Verification items for the finished model (mm, model axes). Face numbers are marked on the shaded views. Give positions to 0.01 mm unless a question says otherwise; leave off trailing zeros. Write each loop counter-clockwise with the first axis right and the second up, starting at its lowest first coordinate (ties: lowest second). Pieces come first, ordered by that corner, then holes.
from build123d import *

# Parameters (mm, degrees)
SKETCH_1_W      = 11
SKETCH_1_H      = 6
SKETCH_1_R      = 1.5
EXTRUDE_1_DEPTH = 2
CHAMFER_1_SIZE  = 1


with BuildPart() as part:
    # Эскиз1 → Бобышка-Вытянуть1 (new body)
    with BuildSketch(Plane(origin=(0, 0, 0), x_dir=(0, 0, -1), z_dir=(1, 0, 0))):
        with Locations((-5.5, 3)):
            Rectangle(SKETCH_1_W, SKETCH_1_H)
        with Locations((-2.5, 3)):
            Circle(SKETCH_1_R, mode=Mode.SUBTRACT)
    extrude(amount=EXTRUDE_1_DEPTH)

    # Фаска1
    chamfer_1_edges = [part.edges().sort_by_distance(p)[0] for p in [
        (0, 3, 4),
    ]]
    chamfer(chamfer_1_edges, length=CHAMFER_1_SIZE - 0.0001)  # a hair under: the kernel refuses the full size


solid = part.part
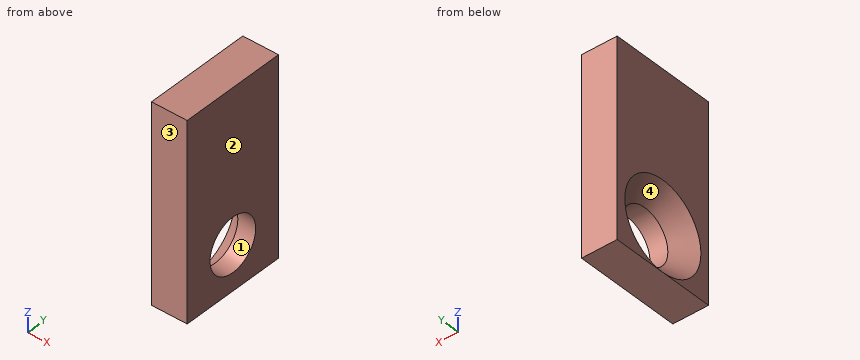
Item 1: Depth check by flat-ended pin: pin 1 (1.8 mm diameter, centred on y = 3, z = 2.5, fed in from +X). Enter the tip coordinate at first touch or a pass-through.
Answer key:
pin 1: passes through
Item 2: Sectioned sample at B-B on z = 2.5. Record the cut outline in (x, y), then the cut area to 3 significant figures.
Answer key:
outline: (0, 0) - (2, 0) - (2, 1.5) - (1, 1.5) - (0, 0.5) - close; (0, 5.5) - (1, 4.5) - (2, 4.5) - (2, 6) - (0, 6) - close
area: 5.00 mm2
Item 3: Sectioned sample at C-C on x = 1.15. Record the cut outline in (y, z), then the cut area to 3 significant figures.
Answer key:
outline: (0, 0) - (6, 0) - (6, 11) - (0, 11) - close; hole circle Ø3 at (3, 2.5)
area: 58.9 mm2
Item 4: Sectioned sample at D-D on x = 0.65. Record the cut outline in (y, z).
Answer key:
outline: (0, 0) - (6, 0) - (6, 11) - (0, 11) - close; hole circle Ø3.7 at (3, 2.5)
Item 5: Release check for a two-part mould opening along Y. For the marked faces 1, 2, 3 and 4 record: released by +Y, released by -Y, zero draft, split by the parting line, or undercut.
Answer key:
face 1: undercut
face 2: zero draft
face 3: released by -Y
face 4: undercut
Item 6: Scan lines: line 1 along Y through (x, z) = (0.5, 2.5); line 2 along Y through (x, z) = (1.75, 2.5); line 3 along Z through (x, y) = (0.7, 4). Record each from-to range of solid material in increasing order.
Answer key:
line 1: y = 0 to 1, 5 to 6
line 2: y = 0 to 1.5, 4.5 to 6
line 3: z = 0 to 1, 4 to 11
